For this review, use the dimensioned drawing (mm, ordinates from the lowest corner) and the shaded views. A direction names the side the tool comes from. Give positions to 0.01 mm unless a question says otherwise; leave off trailing zeros. Write each loop counter-clockwise with the first axis right and the second up, starting at its lowest first coordinate (ties: lowest second). Pieces come first, ordered by that corner, then holes. Notation, with made-up numbers: (12, 47) -> (64, 47) arc R27 ccw to (64, 83) -> close; hole circle Ø9 at (80, 37.5). An arc over 180 degrees is marked (long way). Write each question's results on one line, items separated by ' | '. Start each with the question number.
(1) Take a section at A-A (y = 24). State the section outline as (x, z) points (1 decimal), plus the area to 3 significant figures.
(2) For the marked faces 1, 2 and 3, list the 3-axis set-ups (+Z, -Z, +X, -X, +Y, -Y) from which the entire face can be reached by the end or side of a thin tool; tool diameter is ignored.
(3) Take a section at D-D (y = 31.5). State the section outline as (x, z) points (1 decimal).
(4) Clearance check with flat-ended pins moving along their axes: pin 1 (1.8 mm diameter, centred on y = 10, z = 3, fed in from -X) (1 decimal); pin 2 (3 mm diameter, centred on y = 17.5, z = 21, fed in from +X); pin 3 (13 mm diameter, centred on x = 24.5, y = 24.5, fed in from +Z); pin 4 (12 mm diameter, centred on x = 5.5, y = 43, fed in from +Z). State where each tip first meets the part, or that it passes through.
(5) To check wall thickness, follow probe 1 along Z at (x, y) = (17.75, 34); probe 2 along Y at (x, z) = (24.25, 61.5) (1 decimal); probe 3 along Y at (x, z) = (20.75, 42.5) (1 decimal). State the ranges of each line that lie inside material, in increasing order.
(6) Take a section at B-B (x = 21.5). State the section outline as (y, z) points.
(7) Take a section at C-C (z = 85.5). State the section outline as (x, y) points (1 decimal).
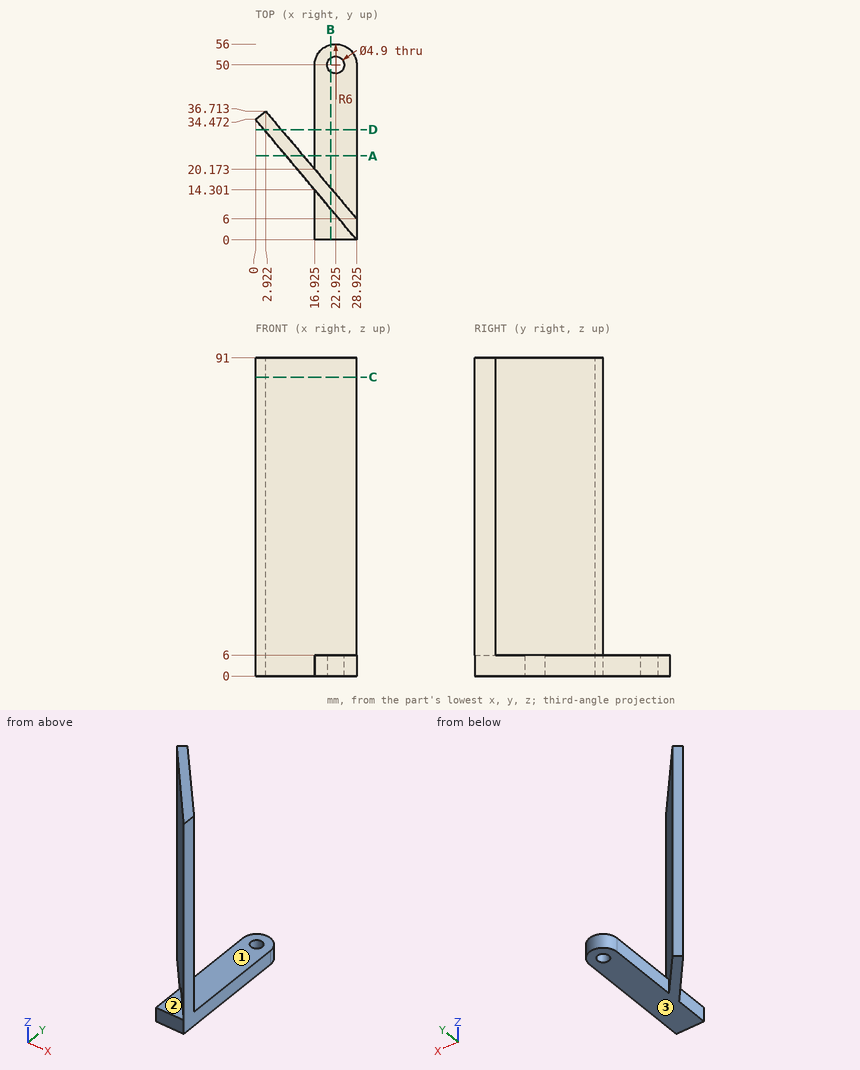
Report:
1) outline: (8.8, 0) -> (13.7, 0) -> (13.7, 91) -> (8.8, 91) -> close; (16.9, 0) -> (28.9, 0) -> (28.9, 6) -> (16.9, 6) -> close | area: 518 mm2
2) face 1: +Z, +X, +Y | face 2: +Z, -X, -Y | face 3: -Z, +X, -X, +Y, -Y
3) outline: (2.5, 0) -> (7.3, 0) -> (7.3, 91) -> (2.5, 91) -> close; (16.9, 0) -> (28.9, 0) -> (28.9, 6) -> (16.9, 6) -> close
4) pin 1: x = 16.9 | pin 2: x = 20.46 | pin 3: z = 6 | pin 4: through
5) probe 1: 0 to 6 | probe 2: 5.6 to 11.5 | probe 3: 9.7 to 15.7
6) outline: (0, 0) -> (48.01, 0) -> (48.01, 6) -> (14.77, 6) -> (14.77, 91) -> (8.85, 91) -> (8.85, 6) -> (0, 6) -> close; (51.99, 0) -> (55.83, 0) -> (55.83, 6) -> (51.99, 6) -> close
7) outline: (0, 34.5) -> (28.9, 0) -> (28.9, 6) -> (2.9, 36.7) -> close
